For this review, take the finished solid that the model builds, in its own axes (mm). A direction names the side the tool comes from. Give positions to 0.01 mm unless a question says otherwise; leave off trailing zeros. Loops run counter-clockwise (first coordinate to the right, second up) from the corner with the lowest first, then second, coordinate; pieces in that order, holes last. Notation, with made-up numbers: (88, -37) - (111, -37) arc R19 cw to (111, -20) - close; hole circle Ø3 at (34, 71). An arc over 180 degrees is marked (long way). Answer in a Markdown table with one row per item.
```python
from build123d import *

# Parameters (mm, degrees)
SKETCH12_R               = 3.4
SKETCH12_R_2             = 1.5
F_30X_30G_X_R1_5_1_DEPTH = 120


with BuildPart() as part:
    # Sketch12 → 铝型材 30X 30G X R1.5(1) (new body)
    with BuildSketch(Plane(origin=(0, 0, 0), x_dir=(0, 0, -1), z_dir=(1, 0, 0))):
        with BuildLine():
            Line((-5.1, 15), (-5.1, 14.5))
            Line((-5.1, 14.5), (-4.1, 14.5))
            Line((-4.1, 14.5), (-4.1, 13.5))
            Line((-4.1, 13.5), (-8.25, 13.5))
            Line((-8.25, 13.5), (-8.25, 9.8))
            Line((-8.25, 9.8), (-4.25, 5.8))
            Line((-4.25, 5.8), (4.25, 5.8))
            Line((4.25, 5.8), (8.25, 9.8))
            Line((8.25, 9.8), (8.25, 13.5))
            Line((8.25, 13.5), (4.1, 13.5))
            Line((4.1, 13.5), (4.1, 14.5))
            Line((4.1, 14.5), (5.1, 14.5))
            Line((5.1, 14.5), (5.1, 15))
            Line((5.1, 15), (13.5, 15))
            ThreePointArc((13.5, 15), (14.560660172, 14.560660172), (15, 13.5))
            Line((15, 13.5), (15, 5.1))
            Line((15, 5.1), (14.5, 5.1))
            Line((14.5, 5.1), (14.5, 4.1))
            Line((14.5, 4.1), (13.5, 4.1))
            Line((13.5, 4.1), (13.5, 8.25))
            Line((13.5, 8.25), (9.8, 8.25))
            Line((9.8, 8.25), (5.8, 4.25))
            Line((5.8, 4.25), (5.8, -4.25))
            Line((5.8, -4.25), (9.8, -8.25))
            Line((9.8, -8.25), (13.5, -8.25))
            Line((13.5, -8.25), (13.5, -4.1))
            Line((13.5, -4.1), (14.5, -4.1))
            Line((14.5, -4.1), (14.5, -5.1))
            Line((14.5, -5.1), (15, -5.1))
            Line((15, -5.1), (15, -13.5))
            ThreePointArc((15, -13.5), (14.560660172, -14.560660172), (13.5, -15))
            Line((13.5, -15), (5.1, -15))
            Line((5.1, -15), (5.1, -14.5))
            Line((5.1, -14.5), (4.1, -14.5))
            Line((4.1, -14.5), (4.1, -13.5))
            Line((4.1, -13.5), (8.25, -13.5))
            Line((8.25, -13.5), (8.25, -9.8))
            Line((8.25, -9.8), (4.25, -5.8))
            Line((4.25, -5.8), (-4.25, -5.8))
            Line((-4.25, -5.8), (-8.25, -9.8))
            Line((-8.25, -9.8), (-8.25, -13.5))
            Line((-8.25, -13.5), (-4.1, -13.5))
            Line((-4.1, -13.5), (-4.1, -14.5))
            Line((-4.1, -14.5), (-5.1, -14.5))
            Line((-5.1, -14.5), (-5.1, -15))
            Line((-5.1, -15), (-13.5, -15))
            ThreePointArc((-13.5, -15), (-14.560660172, -14.560660172), (-15, -13.5))
            Line((-15, -13.5), (-15, -5.1))
            Line((-15, -5.1), (-14.5, -5.1))
            Line((-14.5, -5.1), (-14.5, -4.1))
            Line((-14.5, -4.1), (-13.5, -4.1))
            Line((-13.5, -4.1), (-13.5, -8.25))
            Line((-13.5, -8.25), (-9.8, -8.25))
            Line((-9.8, -8.25), (-5.8, -4.25))
            Line((-5.8, -4.25), (-5.8, 4.25))
            Line((-5.8, 4.25), (-9.8, 8.25))
            Line((-9.8, 8.25), (-13.5, 8.25))
            Line((-13.5, 8.25), (-13.5, 4.1))
            Line((-13.5, 4.1), (-14.5, 4.1))
            Line((-14.5, 4.1), (-14.5, 5.1))
            Line((-14.5, 5.1), (-15, 5.1))
            Line((-15, 5.1), (-15, 13.5))
            ThreePointArc((-15, 13.5), (-14.560660172, 14.560660172), (-13.5, 15))
            Line((-13.5, 15), (-5.1, 15))
        make_face()
        Circle(SKETCH12_R, mode=Mode.SUBTRACT)
        with Locations((-11.5, 11.5)):
            Circle(SKETCH12_R_2, mode=Mode.SUBTRACT)
        with Locations((11.5, 11.5)):
            Circle(SKETCH12_R_2, mode=Mode.SUBTRACT)
        with Locations((-11.5, -11.5)):
            Circle(SKETCH12_R_2, mode=Mode.SUBTRACT)
        with Locations((11.5, -11.5)):
            Circle(SKETCH12_R_2, mode=Mode.SUBTRACT)
    extrude(amount=F_30X_30G_X_R1_5_1_DEPTH)


solid = part.part
```
1. Mouldability with a two-part tool opening along Y and no side actions: class faces 1 (the face through (59, 9, -15)), 2 (the face through (59.16, 11.57, -10)), 3 (the face through (59, -15, 9)) as released by +Y, released by -Y, zero draft, split by the parting line, or undercut.
Values:
| item | result |
|---|---|
| face 1 | zero draft |
| face 2 | undercut |
| face 3 | released by -Y |
2. For faces 4 (the face through (59.16, -7.77, 6.22)), 5 (the face through (0, 0, -4)), list the 3-axis set-ups (+Z, -Z, +X, -X, +Y, -Y) from which the entire face can be reached by the end or side of a thin tool; tool diameter is ignored.
Values:
| item | result |
|---|---|
| face 4 | +X, -X |
| face 5 | +Z, -Z, -X, +Y, -Y |
3. Clearance check with a flat-ended pin moving along its axis: pin 1 (0.5 mm diameter, centred on x = 42.5, y = -14, fed in from -Z). State where the tip first meets the part, or that it passes through.
Values:
| item | result |
|---|---|
| pin 1 | stops at z = -14.98 |
4. We need section C-C, the plane y = 0. Give the boundary of the cut face in (x, z), and give its area (3 significant figures).
Values:
| item | result |
|---|---|
| outline | (0, -5.8) - (120, -5.8) - (120, -3.4) - (0, -3.4) - close; (0, 3.4) - (120, 3.4) - (120, 5.8) - (0, 5.8) - close |
| area | 576 mm^2 |
5. We need section A-A, the plane y = -11.5. Give the boundary of the cut face in (x, z), and give its area (3 significant figures).
Values:
| item | result |
|---|---|
| outline | (0, -15) - (120, -15) - (120, -13) - (0, -13) - close; (0, -10) - (120, -10) - (120, -8.25) - (0, -8.25) - close; (0, 8.25) - (120, 8.25) - (120, 10) - (0, 10) - close; (0, 13) - (120, 13) - (120, 15) - (0, 15) - close |
| area | 900 mm^2 |
6. We need section D-D, the plane x = 7. Count the separate pieces of the cut face and the enclosed holes in it, and give its area (3 significant figures).
Values:
| item | result |
|---|---|
| separate pieces | 1 |
| enclosed holes | 5 |
| area | 336 mm^2 |
7. Wall thickness on line 1 (Y direction, x = 67.5, z = -11.5); line 2 (Y direction, x = 85.5, z = 4.25); line 3 (Y direction, x = 109.5, z = -5.75): over which ranges is each line inside the solid? List them lowest first. Write a range as [from, to].
Values:
| item | result |
|---|---|
| line 1 | y = [-15, -13], [-10, -8.25], [8.25, 10], [13, 15] |
| line 2 | y = [-14.5, -13.5], [-5.8, 5.8], [13.5, 14.5] |
| line 3 | y = [-15, -13.5], [-7.3, 7.3], [13.5, 15] |
